```python
from build123d import *

# Parameters (mm, degrees)
SKETCH1_R               = 25
BOSS_EXTRUDE1_DEPTH     = 10
CUT_EXTRUDE1_DEPTH      = 37.742346142
CUT_EXTRUDE1_DEPTH_BACK = 37.742346142
CUT_EXTRUDE2_DEPTH      = 3
SKETCH5_R               = 2
CUT_EXTRUDE4_DEPTH      = 13
FILLET1_R               = 1
CUT_EXTRUDE6_DEPTH      = 3
CUT_EXTRUDE6_DEPTH_BACK = 3
SKETCH6_W               = 10
SKETCH6_H               = 10


with BuildPart() as part:
    # Sketch1 → Boss-Extrude1 (new body)
    with BuildSketch(Plane.XY):
        Circle(SKETCH1_R)
    extrude(amount=BOSS_EXTRUDE1_DEPTH)

    # Sketch2 → Cut-Extrude1 (cut, two sides: drawn at the far end of the back side and taken through both)
    with BuildSketch(Plane.XY.offset(10).offset(-CUT_EXTRUDE1_DEPTH_BACK)):
        Polygon((5, -5), (15, -5), (15, 5), (5, 5), (5, 15), (-5, 15), (-5, 5), (-15, 5), (-15, -5), (-5, -5), (-5, -15), (5, -15), align=None)
    extrude(amount=CUT_EXTRUDE1_DEPTH + CUT_EXTRUDE1_DEPTH_BACK, mode=Mode.SUBTRACT)

    # Sketch4 → Cut-Extrude2 (cut)
    with BuildSketch(Plane.ZY.offset(-15)):
        Polygon((4.759098318, -4.265594884), (8.57366269, -2.341424419), (8.814564373, 1.924170465), (5.240901682, 4.265594884), (1.42633731, 2.341424419), (1.185435627, -1.924170465), align=None)
    extrude(amount=-CUT_EXTRUDE2_DEPTH, mode=Mode.SUBTRACT)

    # Sketch5 → Cut-Extrude4 (cut)
    with BuildSketch(Plane.ZY.offset(-18)):
        with Locations((5, 0)):
            Circle(SKETCH5_R)
    extrude(amount=-CUT_EXTRUDE4_DEPTH, mode=Mode.SUBTRACT)

    # Fillet1
    fillet1_edges = [part.edges().sort_by_distance(p)[0] for p in [
        (-25, 0, 0),
        (-25, 0, 10),
    ]]
    fillet(fillet1_edges, radius=FILLET1_R)

    # Sketch6 → Cut-Extrude6 (cut, two sides: drawn at the far end of the back side and taken through both)
    with BuildSketch(Plane.YZ.offset(24.999151456).offset(-CUT_EXTRUDE6_DEPTH_BACK)):
        with Locations((0, 5)):
            Rectangle(SKETCH6_W, SKETCH6_H)
    extrude(amount=CUT_EXTRUDE6_DEPTH + CUT_EXTRUDE6_DEPTH_BACK, mode=Mode.SUBTRACT)


solid = part.part
```
The listing builds one solid part. Answer for the finished solid, in the listing's coordinates (mm). A direction names the side the tool comes from. Give positions to 0.01 mm unless a question says otherwise; leave off trailing zeros. Order: outer loops, then holes, each group sorted by start corner. A loop starts at its lowest first (then second) coordinate and runs counter-clockwise, first axis right, second up. Notation, with made-up numbers: (84, 44) - (136, 44) arc R28 cw to (136, 75) - close; hole circle Ø4 at (2, 86). An arc over 180 degrees is marked (long way). Use one line per item in the form item = value. Start each with the question number.
(1) Consider line 1 (Y direction, x = 0, z = 1.5); line 2 (X direction, y = 13, z = 4.25); line 3 (X direction, y = -3, z = 7). Determine where each line is inside the solid, lowest interval first. Write a range as from..to.
(2) Flat-ended cylindrical pins translate along their axes: pin 1 Ø3 at (x, z) = (-11, 5.5) entering from +Y; pin 2 Ø2 at (x, z) = (-8.5, 3.5) entering from -Y; pin 3 Ø5 at (y, z) = (0, 5) entering from +X. Find the tip coordinate at first contact, or state that the pin passes through.
(3) A cutting plane is placed at B-B, the plane y = 0. Write down the section's boundary in (x, z).
(4) The mould has two halves that part along Z. Classify faces 1 (the flat face through (16.479, 0.238, 1.308)), 2 (the flat face through (-6, 6, 10)), 3 (the flat face through (23, -5, 5)): released by +Z, released by -Z, zero draft, split by the parting line, or undercut.
(5) A cutting plane is placed at A-A, the plane x = 0. Write down the section's boundary in (y, z), then the cut area to 3 significant figures.
(6) For faces 4 (the flat face through (5, -10, 5)), 5 (the flat face through (16.479, -3.317, 6.64)), 6 (the cylindrical face through (20, 0, 3)), 7 (the flat face through (23, 5, 5)), determine the directions among +Z, -Z, +X, -X, +Y, -Y from which every point of the face is accessible in a straight line to the end or side of a thin tool.
Ans:
q1.line_1 = -25..-15, 15..25
q1.line_2 = -21.35..-5, 5..21.35
q1.line_3 = -24.82..-15, 18..22
q2.pin_1 = 23.12
q2.pin_2 = -23.85
q2.pin_3 = 22
q3.outline = (-25, 1) arc R1 ccw to (-24, 0) - (-15, 0) - (-15, 10) - (-24, 10) arc R1 ccw to (-25, 9) - close; (15, 0) - (22, 0) - (22, 3) - (18, 3) - (18, 1.29) - (15, 1.29) - close; (15, 8.71) - (18, 8.71) - (18, 7) - (22, 7) - (22, 10) - (15, 10) - close
q4.face_1 = undercut
q4.face_2 = released by +Z
q4.face_3 = zero draft
q5.outline = (-25, 1) arc R1 ccw to (-24, 0) - (-15, 0) - (-15, 10) - (-24, 10) arc R1 ccw to (-25, 9) - close; (15, 0) - (24, 0) arc R1 ccw to (25, 1) - (25, 9) arc R1 ccw to (24, 10) - (15, 10) - close
q5.area = 199 mm^2
q6.face_4 = +Z, -Z
q6.face_5 = none
q6.face_6 = +X
q6.face_7 = +Z, -Z, +X
